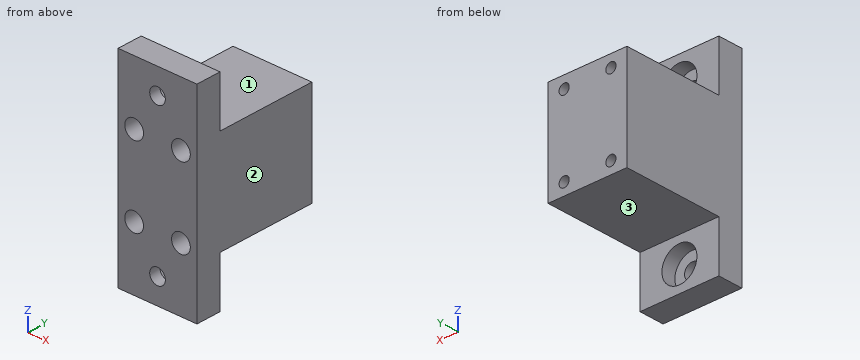
```python
from build123d import *

# Parameters (mm, degrees)
BOSS_EXTRUDE1_DEPTH = 39.99992
SKETCH2_R           = 2.5796875
CUT_EXTRUDE1_DEPTH  = 91.750134452
CUT_EXTRUDE2_START  = -6.35
SKETCH2_3_R         = 4.7625
SKETCH2_3_R_2       = 2.5796875
CUT_EXTRUDE2_DEPTH  = 56.8452
SKETCH3_R           = 3.96875
CUT_EXTRUDE3_DEPTH  = 83.435235239
SKETCH3_5_R         = 8.89
SKETCH3_5_R_2       = 3.96875
CUT_EXTRUDE4_DEPTH  = 7.10438


with BuildPart() as part:
    # Sketch1 → Boss-Extrude1 (new body)
    with BuildSketch(Plane(origin=(0, 0, 0), x_dir=(0, 0, -1), z_dir=(1, 0, 0))):
        Polygon((51.4, 0), (-51.4, 0), (-51.4, 12.6619), (-26, 12.6619), (-26, 63.1952), (26, 63.1952), (26, 12.6619), (51.4, 12.6619), align=None)
    extrude(amount=BOSS_EXTRUDE1_DEPTH)

    # Sketch2 → Cut-Extrude1 (cut, through all)
    with BuildSketch(Plane(origin=(0, 63.1952, 0), x_dir=(1, 0, 0), z_dir=(0, 1, 0))):
        with Locations(Location((8.12496, 19.875, 0), (0, 0, 270))):
            Circle(SKETCH2_R)
        with Locations(Location((31.87496, 19.875, 0), (0, 0, 270))):
            Circle(SKETCH2_R)
        with Locations(Location((8.12496, -19.875, 0), (0, 0, 270))):
            Circle(SKETCH2_R)
        with Locations(Location((31.87496, -19.875, 0), (0, 0, 270))):
            Circle(SKETCH2_R)
    extrude(amount=-CUT_EXTRUDE1_DEPTH, mode=Mode.SUBTRACT)

    # Sketch2<3> → Cut-Extrude2 (cut)
    # profile 1 of 4: a face of its own
    with BuildSketch(Plane(origin=(0, 63.1952, 0), x_dir=(1, 0, 0), z_dir=(0, 1, 0)).offset(CUT_EXTRUDE2_START)):
        with Locations(Location((8.12496, 19.875, 0), (0, 0, 90))):
            Circle(SKETCH2_3_R)
        with Locations(Location((8.12496, 19.875, 0), (0, 0, 270))):
            Circle(SKETCH2_3_R_2, mode=Mode.SUBTRACT)
    # profile 2 of 4: a face of its own
    with BuildSketch(Plane(origin=(0, 63.1952, 0), x_dir=(1, 0, 0), z_dir=(0, 1, 0)).offset(CUT_EXTRUDE2_START)):
        with Locations(Location((31.87496, 19.875, 0), (0, 0, 90))):
            Circle(SKETCH2_3_R)
        with Locations(Location((31.87496, 19.875, 0), (0, 0, 270))):
            Circle(SKETCH2_3_R_2, mode=Mode.SUBTRACT)
    # profile 3 of 4: a face of its own
    with BuildSketch(Plane(origin=(0, 63.1952, 0), x_dir=(1, 0, 0), z_dir=(0, 1, 0)).offset(CUT_EXTRUDE2_START)):
        with Locations(Location((8.12496, -19.875, 0), (0, 0, 90))):
            Circle(SKETCH2_3_R)
        with Locations(Location((8.12496, -19.875, 0), (0, 0, 270))):
            Circle(SKETCH2_3_R_2, mode=Mode.SUBTRACT)
    # profile 4 of 4: a face of its own
    with BuildSketch(Plane(origin=(0, 63.1952, 0), x_dir=(1, 0, 0), z_dir=(0, 1, 0)).offset(CUT_EXTRUDE2_START)):
        with Locations(Location((31.87496, -19.875, 0), (0, 0, 90))):
            Circle(SKETCH2_3_R)
        with Locations(Location((31.87496, -19.875, 0), (0, 0, 270))):
            Circle(SKETCH2_3_R_2, mode=Mode.SUBTRACT)
    extrude(amount=-CUT_EXTRUDE2_DEPTH, mode=Mode.SUBTRACT)

    # Sketch3 → Cut-Extrude3 (cut, through all)
    with BuildSketch(Plane(origin=(0, 12.6619, 0), x_dir=(1, 0, 0), z_dir=(0, 1, 0))):
        with Locations(Location((19.99996, 38.7, 0), (0, 0, 270))):
            Circle(SKETCH3_R)
        with Locations(Location((19.99996, -38.7, 0), (0, 0, 90))):
            Circle(SKETCH3_R)
    extrude(amount=-CUT_EXTRUDE3_DEPTH, mode=Mode.SUBTRACT)

    # Sketch3<5> → Cut-Extrude4 (cut)
    # profile 1 of 2: a face of its own
    with BuildSketch(Plane(origin=(0, 12.6619, 0), x_dir=(1, 0, 0), z_dir=(0, 1, 0))):
        with Locations(Location((19.99996, 38.7, 0), (0, 0, 270))):
            Circle(SKETCH3_5_R)
        with Locations(Location((19.99996, 38.7, 0), (0, 0, 270))):
            Circle(SKETCH3_5_R_2, mode=Mode.SUBTRACT)
    # profile 2 of 2: a face of its own
    with BuildSketch(Plane(origin=(0, 12.6619, 0), x_dir=(1, 0, 0), z_dir=(0, 1, 0))):
        with Locations(Location((19.99996, -38.7, 0), (0, 0, 270))):
            Circle(SKETCH3_5_R)
        with Locations(Location((19.99996, -38.7, 0), (0, 0, 270))):
            Circle(SKETCH3_5_R_2, mode=Mode.SUBTRACT)
    extrude(amount=-CUT_EXTRUDE4_DEPTH, mode=Mode.SUBTRACT)


solid = part.part
```
Design review of the part built by this model. Coordinates are the model's own, in mm. Face numbers are marked on the shaded views. A direction names the side the tool comes from. Give positions to 0.01 mm unless a question says otherwise; leave off trailing zeros. Write each loop counter-clockwise with the first axis right and the second up, starting at its lowest first coordinate (ties: lowest second). Pieces come first, ordered by that corner, then holes.
(1) Add section A-A (z = 38.7). Give the boundary of the cut face in (x, y).
Checked values:
outline: (0, 0) - (16.03, 0) - (16.03, 5.56) - (11.11, 5.56) - (11.11, 12.66) - (0, 12.66) - close; (23.97, 0) - (40, 0) - (40, 12.66) - (28.89, 12.66) - (28.89, 5.56) - (23.97, 5.56) - close
(2) Add section B-B (y = 27). Give the boundary of the cut face in (x, z) (1 decimal), and give its area (3 significant figures).
Checked values:
outline: (0, -26) - (40, -26) - (40, 26) - (0, 26) - close; hole circle Ø9.5 at (8.1, -19.9); hole circle Ø9.5 at (8.1, 19.9); hole circle Ø9.5 at (31.9, -19.9); hole circle Ø9.5 at (31.9, 19.9)
area: 1,790 mm2
(3) Wall thickness on line 1 along X through (y, z) = (54, -20); line 2 along Z through (x, y) = (11, 56.5); line 3 along X through (y, z) = (3.3, -38.7): over which ranges is each line inside the solid? List them lowest first.
Checked values:
line 1: x = 0 to 3.36, 12.89 to 27.11, 36.64 to 40
line 2: z = -26 to -23.67, -16.08 to 16.08, 23.67 to 26
line 3: x = 0 to 16.03, 23.97 to 40
(4) Add section C-C (z = -41). Give the boundary of the cut face in (x, y), and give its area (3 significant figures).
Checked values:
outline: (0, 0) - (16.77, 0) - (16.77, 5.56) - (11.41, 5.56) - (11.41, 12.66) - (0, 12.66) - close; (23.23, 0) - (40, 0) - (40, 12.66) - (28.59, 12.66) - (28.59, 5.56) - (23.23, 5.56) - close
area: 349 mm2
(5) Clearance check with flat-ended pins moving along their axes: pin 1 Ø2 at (x, z) = (8, 37.5) entering from +Y; pin 2 Ø5 at (x, y) = (27.5, 56) entering from +Z. State where each tip first meets the part, or that it passes through.
Checked values:
pin 1: stops at y = 12.66
pin 2: stops at z = 26
(6) Tool access review of the marked faces 1, 2 and 3: name each direction out of +Z, -Z, +X, -X, +Y, -Y from which nothing blocks a thin tool from reaching the whole face with its end or side.
Checked values:
face 1: +Z, +X, -X, +Y
face 2: +Z, -Z, +X, +Y, -Y
face 3: -Z, +X, -X, +Y
